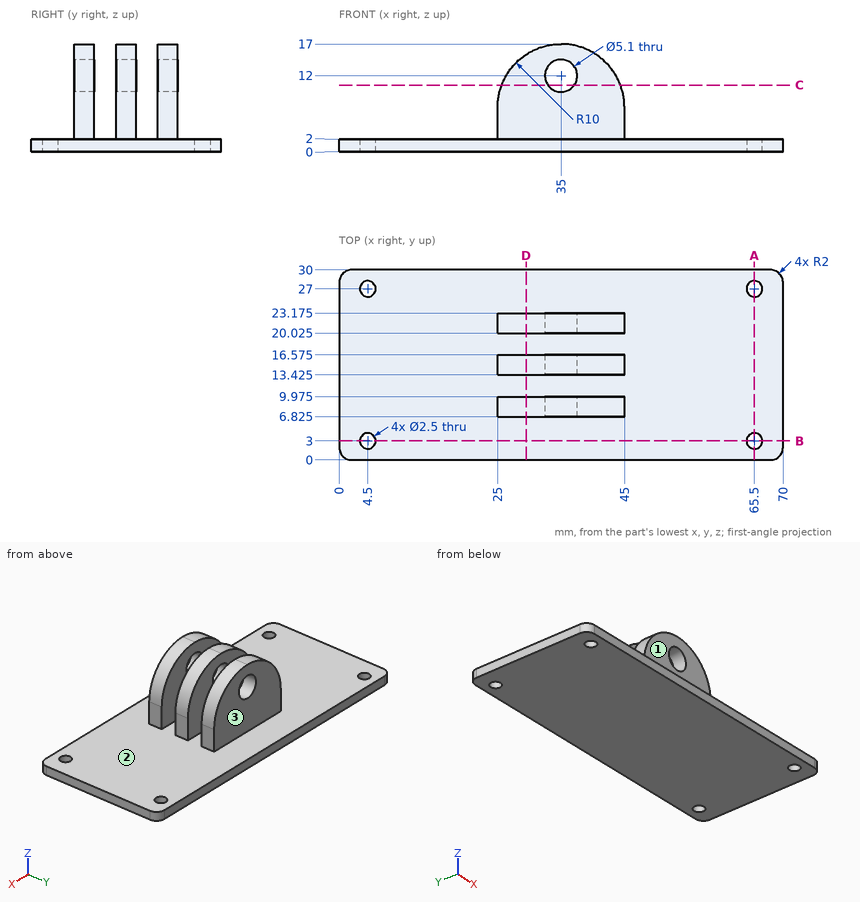
Could you check a few things on this drawing? It's one solid part, dimensions in mm from its lowest x, y, z. A direction names the side the tool comes from. Give positions to 0.01 mm unless a question says otherwise; leave off trailing zeros. Write each loop counter-clockwise with the first axis right and the second up, starting at its lowest first coordinate (ties: lowest second). Pieces come first, ordered by that corner, then holes. Notation, with made-up numbers: (45.25, -23) -> (63.25, -23) arc R19 cw to (63.25, 12) -> close; hole circle Ø9 at (-26.75, 43). An arc over 180 degrees is marked (long way). Answer as CSV lines item,"result". Start each with the question number.
(1) Which directions (+Z, -Z, +X, -X, +Y, -Y) give clear straight access to the entire face, cutting with the end or side of a thin tool? Please do the marked faces 1, 2 and 3.
(2) If we section it at B-B, the plane y = 3: Write out the boundary of the cut face in (x, z), and give its area (3 significant figures).
(3) I'm going to push flat-ended pins straight in: pin 1 Ø3.5 at (y, z) = (15, 3.5) entering from +X; pin 2 Ø1.5 at (x, y) = (34.5, 6) entering from +Z; pin 3 Ø6 at (x, z) = (35, 12) entering from -Y (3 decimals); pin 4 Ø9 at (x, y) = (45.5, 14) entering from +Z. Where does each tip first touch, or does it pass through?
(4) Please list where these lines run through material, in increasing order: line 1 (Y direction, x = 42.5, z = 2.5) (3 decimals); line 2 (Y direction, x = 4.5, z = 0.85); line 3 (Z direction, x = 35, y = 14.45).
(5) If we section it at D-D, the plane x = 29.5: Write out the boundary of the cut face in (y, z) (3 decimals), and give its area (3 significant figures).
(6) If we section it at A-A, the plane x = 65.5: Write out the boundary of the cut face in (y, z).
(7) If we section it at C-C, the plane z = 10.5: Write out the boundary of the cut face in (x, y) (1 decimal).
Answer list:
1,face 1,"+Z, +X, -X, -Y"
1,face 2,"+Z"
1,face 3,"+Z, +X, -X, +Y"
2,outline,"(0, 0) -> (3.25, 0) -> (3.25, 2) -> (0, 2) -> close; (5.75, 0) -> (64.25, 0) -> (64.25, 2) -> (5.75, 2) -> close; (66.75, 0) -> (70, 0) -> (70, 2) -> (66.75, 2) -> close"
2,area,"130 mm^2"
3,pin 1,"x = 70"
3,pin 2,"z = 2"
3,pin 3,"y = 6.825"
3,pin 4,"z = 15"
4,line 1,"6.825 to 9.975, 13.425 to 16.575, 20.025 to 23.175"
4,line 2,"0 to 1.75, 4.25 to 25.75, 28.25 to 30"
4,line 3,"0 to 9.45, 14.55 to 17"
5,outline,"(0, 0) -> (30, 0) -> (30, 2) -> (23.175, 2) -> (23.175, 15.352) -> (20.025, 15.352) -> (20.025, 2) -> (16.575, 2) -> (16.575, 15.352) -> (13.425, 15.352) -> (13.425, 2) -> (9.975, 2) -> (9.975, 15.352) -> (6.825, 15.352) -> (6.825, 2) -> (0, 2) -> close"
5,area,"186 mm^2"
6,outline,"(0, 0) -> (1.75, 0) -> (1.75, 2) -> (0, 2) -> close; (4.25, 0) -> (25.75, 0) -> (25.75, 2) -> (4.25, 2) -> close; (28.25, 0) -> (30, 0) -> (30, 2) -> (28.25, 2) -> close"
7,outline,"(25.6, 6.8) -> (32.9, 6.8) -> (32.9, 10) -> (25.6, 10) -> close; (25.6, 13.4) -> (32.9, 13.4) -> (32.9, 16.6) -> (25.6, 16.6) -> close; (25.6, 20) -> (32.9, 20) -> (32.9, 23.2) -> (25.6, 23.2) -> close; (37.1, 6.8) -> (44.4, 6.8) -> (44.4, 10) -> (37.1, 10) -> close; (37.1, 13.4) -> (44.4, 13.4) -> (44.4, 16.6) -> (37.1, 16.6) -> close; (37.1, 20) -> (44.4, 20) -> (44.4, 23.2) -> (37.1, 23.2) -> close"
